Geometry: see drawing. Coordinates: mm, zero at the bounding-box minimum. A direction names the side the tool comes from. Coordinates: 2 decimals unless noted, no trailing zeros. Order: outer loops, then holes, each group sorted by start corner. A loop starts at its lowest first (then second) coordinate and runs counter-clockwise, first axis right, second up. Notation, with made-up numbers: (-28.5, -10.5) -> (-14.5, -10.5) arc R32 cw to (-14.5, 19.5) -> close; hole circle Ø6 at (29.25, 13). An arc over 180 degrees is marked (long way). Write each question's results on one line, items separated by ' | '.
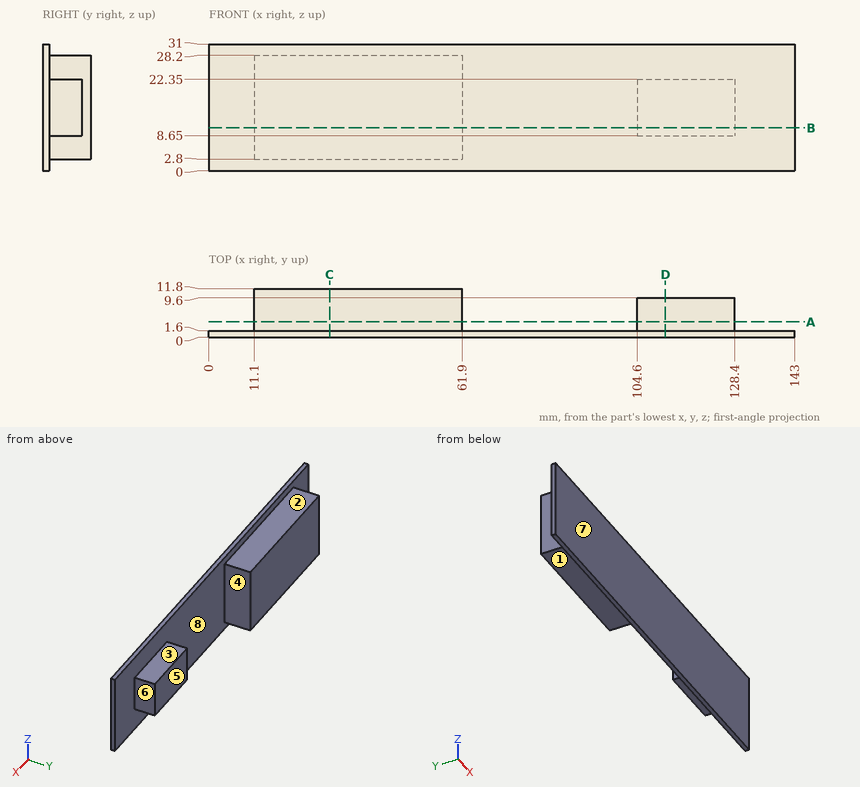
(1) Line query: line 1 along X through (y, z) = (6, 14); line 2 along Y through (x, z) = (120.5, 18); line 3 along Y through (x, z) = (81.5, 2.5). Output: solid intervals per line, ascending. Write a range as from..to.
Return value:
line 1: 11.1..61.9, 104.6..128.4 | line 2: 0..9.6 | line 3: 0..1.6
(2) Pin query (flat end, axial travel): P1, Ø6, axis at x = 121.5, y = 3.5, coming from the +Z side; P2, Ø2, axis at y = 9, z = 18.5, coming from the +X side; P3, Ø4, axis at x = 118.5, z = 14, coming from the +Y side; P4, Ø2.5, axis at x = 122.5, y = 4.5, coming from the -Z side. Return the tip coordinate at first contact, or that it passes through.
Return value:
P1: z = 31 | P2: x = 128.4 | P3: y = 9.6 | P4: z = 8.65
(3) Reachability of the marked faces 1, 2, 3, 4 and 5 from +Z, -Z, +X, -X, +Y, -Y: full face, straight path, thin tool, end or side. Return the list, or none.
Return value:
face 1: -Z, +X, -X, +Y | face 2: +Z, +X, -X, +Y | face 3: +Z, +X, +Y | face 4: +Z, -Z, +Y | face 5: +Z, -Z, +X, +Y
(4) Cut plane B-B, the plane z = 10.5. Return loops of the section in (x, y).
Return value:
outline: (0, 0) -> (143, 0) -> (143, 1.6) -> (128.4, 1.6) -> (128.4, 9.6) -> (104.6, 9.6) -> (104.6, 1.6) -> (61.9, 1.6) -> (61.9, 11.8) -> (11.1, 11.8) -> (11.1, 1.6) -> (0, 1.6) -> close
(5) Mould query, pull axis X, two halves, no side actions, for the marked faces 6, 7 and 8. Classes: +X half, -X half, draft (parallel to the pull), parting line (faces both ways), or undercut.
Return value:
face 6: +X half | face 7: draft | face 8: undercut
(6) Cut plane D-D, the plane x = 111.5. Return loops of the section in (y, z).
Return value:
outline: (0, 0) -> (1.6, 0) -> (1.6, 8.65) -> (9.6, 8.65) -> (9.6, 22.35) -> (1.6, 22.35) -> (1.6, 31) -> (0, 31) -> close
(7) Cut plane A-A, the plane y = 3.75. Return loops of the section in (x, z), plus the area to 3 significant figures.
Return value:
outline: (11.1, 2.8) -> (61.9, 2.8) -> (61.9, 28.2) -> (11.1, 28.2) -> close; (104.6, 8.65) -> (128.4, 8.65) -> (128.4, 22.35) -> (104.6, 22.35) -> close | area: 1,620 mm2
(8) Cut plane C-C, the plane x = 29.5. Return loops of the section in (y, z), plus the area to 3 significant figures.
Return value:
outline: (0, 0) -> (1.6, 0) -> (1.6, 2.8) -> (11.8, 2.8) -> (11.8, 28.2) -> (1.6, 28.2) -> (1.6, 31) -> (0, 31) -> close | area: 309 mm2
